```python
from build123d import *

# Parameters (mm, degrees)
SKETCH_1_W      = 15
SKETCH_1_H      = 8
EXTRUDE_1_DEPTH = 20


with BuildPart() as part:
    # 草图1 → 凸台-拉伸1 (new body)
    with BuildSketch(Plane(origin=(0, 0, 0), x_dir=(1, 0, 0), z_dir=(0, 1, 0))):
        with Locations((7.5, 4)):
            Rectangle(SKETCH_1_W, SKETCH_1_H)
        with BuildLine():
            Line((8.763068312, 1.6), (11.236931688, 1.6))
            ThreePointArc((11.236931688, 1.6), (10, 6.7), (8.763068312, 1.6))
        make_face(mode=Mode.SUBTRACT)
    extrude(amount=EXTRUDE_1_DEPTH)


solid = part.part
```
The model under review builds one solid part; all positions refer to its coordinate system, in mm. A direction names the side the tool comes from. Round coordinates to 2 decimals unless told otherwise and drop trailing zeros. Loops run counter-clockwise (first coordinate to the right, second up) from the corner with the lowest first, then second, coordinate; pieces in that order, holes last.
1) Clearance check with a flat-ended pin moving along its axis: P1, Ø4, axis at y = 6.5, z = -7, coming from the -X side. State where the tip first meets the part, or that it passes through.
Values follow:
P1: stops at x = 0
2) Consider section A-A on z = -4. State the section outline as (x, y) points, then the cut area to 3 significant figures.
Values follow:
outline: (0, 0) - (7.3, 0) - (7.3, 20) - (0, 20) - close; (12.7, 0) - (15, 0) - (15, 20) - (12.7, 20) - close
area: 192 mm2
3) Wall thickness on line 1 along Z through (x, y) = (10, 9.25); line 2 along X through (y, z) = (11.5, -4); line 3 along X through (y, z) = (10.25, -1.75): over which ranges is each line inside the solid? List them lowest first.
Values follow:
line 1: z = -8 to -6.7, -1.6 to 0
line 2: x = 0 to 7.3, 12.7 to 15
line 3: x = 0 to 8.51, 11.49 to 15
4) The part is to be moulded in two halves that separate along Z. For faces 1 (the face through (10.1, 9.9, -6.7)), 2 (the face through (7, 10, 0)), 3 (the face through (6, 0, -4)), say which applies: pulls with the +Z half, pulls with the -Z half, needs draft (parallel to the pull), parting line crosses it, or undercut.
Values follow:
face 1: undercut
face 2: pulls with the +Z half
face 3: needs draft
5) Consider section C-C on y = 17. State the section outline as (x, z) points, then the cut area to 3 significant figures.
Values follow:
outline: (0, -8) - (15, -8) - (15, 0) - (0, 0) - close; hole (8.76, -1.6) arc R2.7 ccw (long way) to (11.24, -1.6) - close
area: 97.6 mm2
6) Tool access review of faces 4 (the face through (10, 10, -1.6)), 5 (the face through (7, 10, -8)): name each direction out of +Z, -Z, +X, -X, +Y, -Y from which nothing blocks a thin tool from reaching the whole face with its end or side.
Values follow:
face 4: +Y, -Y
face 5: -Z, +X, -X, +Y, -Y
7) Consider section B-B on x = 10. State the section outline as (y, z) points.
Values follow:
outline: (0, -8) - (20, -8) - (20, -6.7) - (0, -6.7) - close; (0, -1.6) - (20, -1.6) - (20, 0) - (0, 0) - close
